Can you work these out from the model? Positions are in its coordinate system, mm. Face numbers are marked on the shaded views. Coordinates: 2 decimals unless noted, no trailing zeros. Order: outer loops, then holes, each group sorted by start corner. A loop starts at its lowest first (then second) coordinate and runs counter-clockwise, first axis right, second up.
Autodesk Inventor part; units mm, degrees
ref_plane "YZ Plane" through (0, 0, 0) normal (1, 0, 0) x (0, 1, 0)
ref_plane "XZ Plane" through (0, 0, 0) normal (0, 1, 0) x (-1, 0, 0)
ref_plane "XY Plane" through (0, 0, 0) normal (0, 0, 1) x (1, 0, 0)
sketch "Sketch1" plane through (0, 0, 0) normal (0, 0, 1) x (1, 0, 0)
  line L0 (50.8, 0) -> (50.8, 39.0312) construction
  line L1 (0, 0) -> (50.6412, 0)
  line L2 (44.45, 0) -> (44.45, 51.6727)
  line L3 (0, 0) -> (0, 50.5742)
  line L4 (50.6412, 0) -> (50.6412, 45.6895)
  line L5 (50.6412, 4.7625) -> (44.45, 4.7625)
  line L6 (44.45, 11.1125) -> (50.6412, 11.1125)
  line L7 (50.6412, 30.1625) -> (44.45, 30.1625)
  line L8 (44.45, 36.5125) -> (50.6412, 36.5125)
  line L9 (50.6412, 41.275) -> (0, 41.275)
  point P0 (47.5456, 36.5125)
  point P1 (44.45, 30.1625)
  dimension "d1" = 50.6412
  dimension "d2" = 44.45
  dimension "d3" = 6.35
  dimension "d4" = 6.35
  dimension "d5" = 4.7625
  dimension "d6" = 19.05
  dimension "d7" = 4.7625
  dimension "d12" = 41.275
revolve "Revolution1" add sketch "Sketch1" angle 360 about axis through (0, 0, 0) along (0, 1, 0) contours L3 L9 L2 L1 | L2 L5 L4 L1 | L9 L4 L8 L2 | L2 L7 L4 L6
chamfer "Chamfer1" distance 0.635 angle 45 6 edges at (-50.6412, 0, 0) (-50.6412, 4.7625, 0) (-50.6412, 11.1125, 0) (-50.6412, 30.1625, 0) (-50.6412, 36.5125, 0) (-50.6412, 41.275, 0)
sketch "Sketch2" plane through (0, 0, 0) normal (0, -1, 0) x (1, 0, 0)
  circle A0 centre (0, 0) radius 9.7409
  circle A1 centre (0, 0) radius 11.1125
  dimension "d16" = 19.4818
  dimension "d17" = 22.225
extrude "Extrusion1" cut sketch "Sketch2" against normal up to surface (30.1625 mm away) contours A0
extrude "Extrusion2" cut sketch "Sketch2" against normal blind 6.35 contours A0 | A1
equation "\"MachineMaxHeight\" = 539.75"
equation "\"MachineMaxWidth\" = 215.9"
equation "\"MachineMaxLength\" = 266.7"
equation "\"MachineFluidCapacity\" = 25.4"
equation "\"MaxCompressiveCapacity\" = 20320"
equation "\"WashChamberID\" = 101.6"
equation "\"WashChamberOD\" = 114.3"
equation "\"ConduitThickness\" = 152.4"
equation "\"SealedSurfaceOffset\" = 0.15875"
equation "\"StaticORingThickness\" = 4.7625"
properties part number "2 Piston"
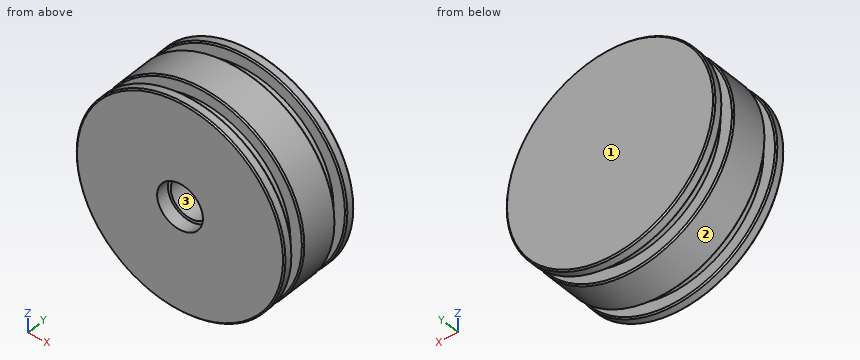
1. Imagine slicing it at B-B on y = 32. Please give me the cut outline in (x, z).
Completed:
outline: circle Ø88.9 at (0, 0)
2. I'm going to push flat-ended pins straight in: pin 1 (2 mm diameter, centred on x = 11.5, y = 8, fed in from +Z); pin 2 (12 mm diameter, centred on x = 22.5, y = 27.5, fed in from +Z); pin 3 (5 mm diameter, centred on x = -39.5, y = 29, fed in from +Z). Where does each tip first touch, or does it pass through?
Completed:
pin 1: stops at z = 43.19
pin 2: stops at z = 47.88
pin 3: stops at z = 34.58
3. Please list where these lines run through material, in increasing order: probe 1 along Y at (x, z) = (42.5, -27); probe 2 along Z at (x, y) = (0, 4); probe 3 along Z at (x, y) = (-1, 30).
Completed:
probe 1: y = 0.35 to 4.42, 11.46 to 29.82, 36.86 to 40.93
probe 2: z = -50.64 to -11.11, 11.11 to 50.64
probe 3: z = -50.16 to -9.69, 9.69 to 50.16
4. Thinking about a two-plate mould opening in X: for the marked faces 1, 2 and 3, which applies, pulls with the +X half, pulls with the -X half, needs draft (parallel to the pull), parting line crosses it, or undercut?
Completed:
face 1: needs draft
face 2: parting line crosses it
face 3: undercut
5. Imagine slicing it at A-A on y = 8. Please give me the cut outline in (x, z), then the cut area to 3 significant figures.
Completed:
outline: circle Ø88.9 at (0, 0); hole circle Ø19.48 at (0, 0)
area: 5,910 mm2
